```python
from build123d import *

# Parameters (mm, degrees)
BASE_EXTRUDE_DEPTH = 12
SKETCH4_R          = 3
PIVOTPIN_DEPTH     = 15
M5_X_0_8_1_D       = 4.2
M5_X_0_8_1_DEPTH   = 12
M5_X_0_8_1_TIP     = 1.2618073
M5_DRILLED2_D      = 4.2
M5_DRILLED2_DEPTH  = 12
M5_DRILLED2_TIP    = 1.2618073


with BuildPart() as part:
    # Sketch3 → Base-Extrude (new body)
    with BuildSketch(Plane.XY):
        with BuildLine():
            Line((-15.5, 0), (0, 0))
            Line((0, 0), (0, 48))
            Line((0, 48), (-10, 48))
            Line((-10, 48), (-10, 11.979130372))
            ThreePointArc((-10, 11.979130372), (-13.915880433, 10.062019202), (-15.5, 6))
            Line((-15.5, 6), (-15.5, 0))
        make_face()
    extrude(amount=BASE_EXTRUDE_DEPTH)

    # Sketch4 → PivotPin (add, symmetric)
    with BuildSketch(Plane.XY.offset(6)):
        with Locations(Location((-5, 3, 0), (0, 0, 270))):
            Circle(SKETCH4_R)
    extrude(amount=PIVOTPIN_DEPTH, both=True)

    # M5 x 0.8 #1
    with Locations(Plane(origin=(-10, -42.79947187, 57.720392954), x_dir=(0, 0, 1), z_dir=(-1, 0, 0))):
        with Locations((-51.720392954, 84.79947187)):
            Hole(M5_X_0_8_1_D / 2, depth=M5_X_0_8_1_DEPTH)
            with Locations((0, 0, -(M5_X_0_8_1_DEPTH + M5_X_0_8_1_TIP / 2))):  # 118° drill point
                Cone(0, M5_X_0_8_1_D / 2, M5_X_0_8_1_TIP, mode=Mode.SUBTRACT)

    # M5 Drilled2
    with Locations(Plane(origin=(-10, -44.641735567, 57.583928977), x_dir=(0, 0, 1), z_dir=(-1, 0, 0))):
        with Locations((-51.583928977, 74.641735567)):
            Hole(M5_DRILLED2_D / 2, depth=M5_DRILLED2_DEPTH)
            with Locations((0, 0, -(M5_DRILLED2_DEPTH + M5_DRILLED2_TIP / 2))):  # 118° drill point
                Cone(0, M5_DRILLED2_D / 2, M5_DRILLED2_TIP, mode=Mode.SUBTRACT)


solid = part.part
```
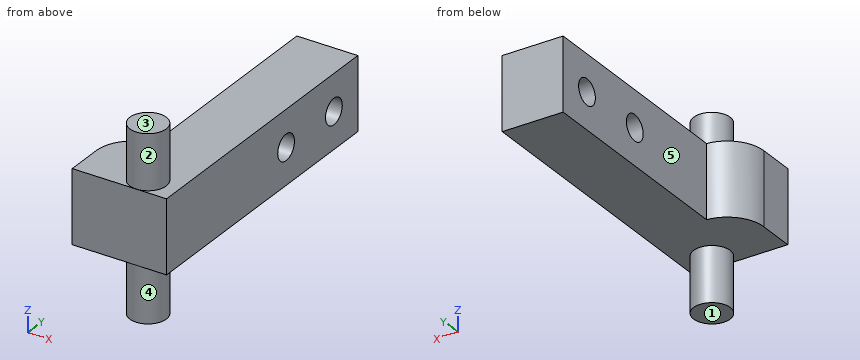
Model file for the job. Use its own axes, mm. Face numbers are marked on the shaded views. A direction names the side the tool comes from. Give positions to 0.01 mm unless a question says otherwise; leave off trailing zeros. Order: outer loops, then holes, each group sorted by start corner. A loop starts at its lowest first (then second) coordinate and runs counter-clockwise, first axis right, second up.
1) Saw through at A-A, the plane y = 42. Write the cut outline in (x, z), then the cut area to 3 significant figures.
2) Saw through at C-C, the plane x = -9.25. Write the cut outline in (y, z), then the cut area to 3 significant figures.
3) Wall check: probe 1 along Y at (x, z) = (-3, 6); probe 2 along Y at (x, z) = (-6.25, 7.5); probe 3 along Z at (x, y) = (-1.5, 27.5). Give the ranges that are in metal, low to high.
4) Pin check, flat tips, straight feed: pin 1 (4.5 mm diameter, centred on x = -5, y = 31, fed in from +Z); pin 2 (6 mm diameter, centred on y = 30.5, z = 3.5, fed in from -X); pin 3 (4 mm diameter, centred on x = -8, y = 35, fed in from -Z). Stop position of each tip, or through.
5) 3-axis set-ups, long thin cutter, end or side, ignore diameter. For the marked faces 1, 2, 3, 4 and 5: which of +Z, -Z, +X, -X, +Y, -Y reach the whole face in a straight line?
6) Saw through at B-B, the plane z = 6. Write the cut outline in (x, y).
7) Saw through at D-D, the plane y = 3. Write the cut outline in (x, z), then the cut area to 3 significant figures.
Computed:
1. outline: (-10, 0) - (0, 0) - (0, 3.9) - (-10, 3.9) - close; (-10, 8.1) - (0, 8.1) - (0, 12) - (-10, 12) - close
1. area: 78.0 mm2
2. outline: (0, 0) - (48, 0) - (48, 12) - (0, 12) - close; hole circle Ø4.2 at (30, 6); hole circle Ø4.2 at (42, 6)
2. area: 548 mm2
3. probe 1: y = 0 to 27.9, 32.1 to 39.9, 44.1 to 48
3. probe 2: y = 0 to 28.53, 31.47 to 40.53, 43.47 to 48
3. probe 3: z = 0 to 12
4. pin 1: stops at z = 12
4. pin 2: stops at x = -10
4. pin 3: stops at z = 0
5. face 1: -Z, +X, -X, +Y, -Y
5. face 2: +Z
5. face 3: +Z, +X, -X, +Y, -Y
5. face 4: -Z
5. face 5: +Z, -Z, -X, +Y
6. outline: (-15.5, 0) - (0, 0) - (0, 27.9) - (-10, 27.9) - (-10, 11.98) arc R6 ccw to (-15.5, 6) - close; (-10, 32.1) - (0, 32.1) - (0, 39.9) - (-10, 39.9) - close; (-10, 44.1) - (0, 44.1) - (0, 48) - (-10, 48) - close
7. outline: (-15.5, 0) - (-8, 0) - (-8, -9) - (-2, -9) - (-2, 0) - (0, 0) - (0, 12) - (-2, 12) - (-2, 21) - (-8, 21) - (-8, 12) - (-15.5, 12) - close
7. area: 294 mm2
